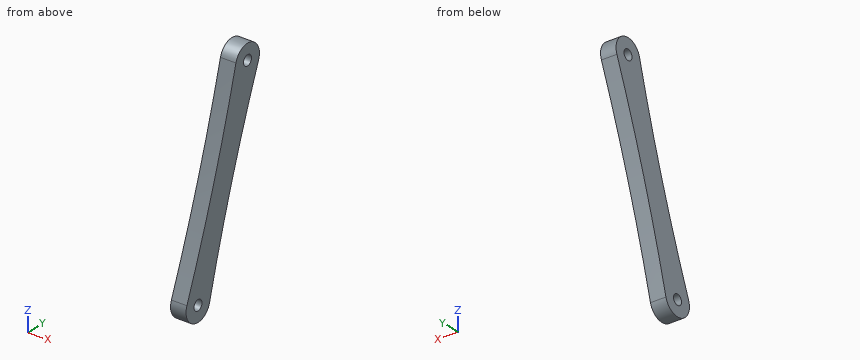
```python
from build123d import *

# Parameters (mm, degrees)
SKETCH2_R               = 1
BOSS_EXTRUDE2_DEPTH     = 3
SCALE1_SCALE            = 2
CUT_EXTRUDE1_DEPTH      = 166.58723061
CUT_EXTRUDE1_DEPTH_BACK = 166.58723061


with BuildPart() as part:
    # Sketch2 → Boss-Extrude2 (new body)
    with BuildSketch(Plane.YZ):
        with BuildLine():
            ThreePointArc((19.533132157, 81.629722684), (24.352585485, 66.108442404), (37.508583242, 75.650821296))
            ThreePointArc((37.508583242, 75.650821296), (40.136593734, 92.158254486), (47.919515666, 106.951087747))
            ThreePointArc((47.919515666, 106.951087747), (43.100062338, 122.472368027), (29.944064581, 112.929989135))
            ThreePointArc((29.944064581, 112.929989135), (27.316054088, 96.422555945), (19.533132157, 81.629722684))
        make_face()
        with Locations(Location((39.943921454, 112.983491659, 0), (0, 0, 270))):
            Circle(SKETCH2_R, mode=Mode.SUBTRACT)
        with Locations(Location((27.508726369, 75.597318771, 0), (0, 0, 270))):
            Circle(SKETCH2_R, mode=Mode.SUBTRACT)
    extrude(amount=BOSS_EXTRUDE2_DEPTH)


with BuildPart() as part_1:
    # Scale1: scaled about (1.5, 33.726323911, 94.290405215)
    add(part.part.scale(SCALE1_SCALE).moved(Location((-1.5, -33.726323911, -94.290405215))))

    # Sketch3 → Cut-Extrude1 (cut, two sides: drawn at the far end of the back side and taken through both)
    # profile 1 of 2: a face of its own
    with BuildSketch(Plane.YZ.offset(4.5).offset(-CUT_EXTRUDE1_DEPTH_BACK)):
        with BuildLine():
            ThreePointArc((70.088301632, 113.579366365), (56.035739925, 86.869962872), (51.290699446, 57.064739901))
            ThreePointArc((51.290699446, 57.064739901), (11.822706174, 28.437603225), (-2.635653809, 75.001444065))
            ThreePointArc((-2.635653809, 75.001444065), (11.416907898, 101.710847558), (16.161948377, 131.516070529))
            ThreePointArc((16.161948377, 131.516070529), (55.629941649, 160.143207206), (70.088301632, 113.579366365))
        make_face()
        with BuildLine():
            ThreePointArc((26.16180525, 131.569573054), (20.905784266, 98.554706674), (5.339940403, 68.969040153))
            ThreePointArc((5.339940403, 68.969040153), (14.978847058, 37.926479592), (41.290842573, 57.011237377))
            ThreePointArc((41.290842573, 57.011237377), (46.546863557, 90.026103756), (62.11270742, 119.611770278))
            ThreePointArc((62.11270742, 119.611770278), (52.473800765, 150.654330838), (26.16180525, 131.569573054))
        make_face(mode=Mode.SUBTRACT)
    # profile 2 of 2: a face of its own
    with BuildSketch(Plane.YZ.offset(4.5).offset(-CUT_EXTRUDE1_DEPTH_BACK)):
        with BuildLine():
            ThreePointArc((62.11270742, 119.611770278), (52.473800765, 150.654330838), (26.16180525, 131.569573054))
            ThreePointArc((26.16180525, 131.569573054), (20.905784266, 98.554706674), (5.339940403, 68.969040153))
            ThreePointArc((5.339940403, 68.969040153), (14.978847058, 37.926479592), (41.290842573, 57.011237377))
            ThreePointArc((41.290842573, 57.011237377), (46.546863557, 90.026103756), (62.11270742, 119.611770278))
        make_face()
        with BuildLine():
            ThreePointArc((15.723577438, 59.140830534), (19.398551743, 51.210538273), (27.089730835, 55.362734759))
            ThreePointArc((27.089730835, 55.362734759), (38.273895697, 92.777815454), (51.72819988, 129.437814172))
            ThreePointArc((51.72819988, 129.437814172), (48.056310902, 137.369535475), (40.363517101, 133.220331331))
            ThreePointArc((40.363517101, 133.220331331), (29.171473339, 95.805416009), (15.723577438, 59.140830534))
        make_face(mode=Mode.SUBTRACT)
    extrude(amount=CUT_EXTRUDE1_DEPTH + CUT_EXTRUDE1_DEPTH_BACK, mode=Mode.SUBTRACT)


solid = part_1.part
```
Geometry check sheet. Reference: the model listing, model coordinates, mm. Round coordinates to 2 decimals unless told otherwise and drop trailing zeros. Order: outer loops, then holes, each group sorted by start corner. A loop starts at its lowest first (then second) coordinate and runs counter-clockwise, first axis right, second up. Notation, with made-up numbers: (-33.5, -8) -> (-22.5, -8) arc R11 cw to (-22.5, 12) -> close; hole circle Ø6 at (66.5, -32). An arc over 180 degrees is marked (long way). Return JSON: item names as keys, results as strings. Group by question number.
Q1. Section check D-D, the plane y = 33.5. Record the boundary of the cut face in (x, z).
Q2. Section check C-C, the plane z = 74. Record the boundary of the cut face in (x, y), plus the area to 3 significant figures.
Q3. Section check B-B, the plane x = 0.8. Record the boundary of the cut face in (y, z), plus the area to 3 significant figures.
Q4. Section check A-A, the plane y = 22.5. Record the boundary of the cut face in (x, z), plus the area to 3 significant figures.
Q5. Gauge pin test, flat ends, axial feed: pin 1 (3 mm diameter, centred on x = 1.5, z = 127, fed in from +Y); pin 2 (3 mm diameter, centred on x = 3.5, z = 69, fed in from +Y); pin 3 (3 mm diameter, centred on x = -0.5, z = 93.5, fed in from +Y). Record the tip position at first contact, or that the pin passes through.
Q6. Material ranges on probe 1 along Y at (x, z) = (1.8, 56); probe 2 along Y at (x, z) = (0.2, 70); probe 3 along Y at (x, z) = (0.05, 125.5), recorded low to high. Write a range as from..to.
Numbers:
{
 "1": {"outline": "(-1.5, 77.81) -> (4.5, 77.81) -> (4.5, 109.32) -> (-1.5, 109.32) -> close"},
 "2": {"outline": "(-1.5, 21.48) -> (4.5, 21.48) -> (4.5, 32.35) -> (-1.5, 32.35) -> close", "area": "65.2 mm^2"},
 "3": {"outline": "(15.72, 59.14) arc R6 ccw (long way) to (27.09, 55.36) arc R637.42 cw to (51.73, 129.44) arc R6 ccw (long way) to (40.36, 133.22) arc R641.52 cw to start; hole circle Ø4 at (21.29, 56.9); hole circle Ø4 at (46.16, 131.68)", "area": "908 mm^2"},
 "4": {"outline": "(-1.5, 51.03) -> (4.5, 51.03) -> (4.5, 55.31) -> (-1.5, 55.31) -> close; (-1.5, 58.5) -> (4.5, 58.5) -> (4.5, 76.75) -> (-1.5, 76.75) -> close", "area": "135 mm^2"},
 "5": {"pin 1": "y = 51.35", "pin 2": "y = 31.31", "pin 3": "y = 39.02"},
 "6": {"probe 1": "15.36..19.51, 23.08..27.26", "probe 2": "19.97..31.17", "probe 3": "38.26..50.16"}
}
